Input: part model. Units: mm. Frame: model coordinates. A direction names the side the tool comes from. Coordinates: 2 decimals unless noted, no trailing zeros. Loops run counter-clockwise (first coordinate to the right, second up) from the corner with the lowest first, then second, coordinate; pieces in that order, holes last.
```python
from build123d import *

# Parameters (mm, degrees)
SKETCH_1_W          = 136
SKETCH_1_H          = 104
EXTRUDE_1_DEPTH     = 42
SKETCH_2_W          = 130
SKETCH_2_H          = 98
CUT_EXTRUDE_1_DEPTH = 36
CUT_EXTRUDE_2_REACH = 94.865
SKETCH_3_R          = 5
SKETCH_4_R          = 5
CUT_EXTRUDE_3_DEPTH = 136
SKETCH_5_R          = 5
CUT_EXTRUDE_4_DEPTH = 104
SKETCH_6_W          = 3
SKETCH_6_H          = 20
EXTRUDE_2_DEPTH     = 100
SKETCH_7_R          = 10
EXTRUDE_3_DEPTH     = 130
EXTRUDE_4_DEPTH     = 3
EXTRUDE_START       = -3
EXTRUDE_5_DEPTH     = 3
SKETCH_10_W         = 1.2
SKETCH_10_H         = 2
CUT_EXTRUDE_5_DEPTH = 104
SKETCH_11_W         = 1.2
SKETCH_11_H         = 2
CUT_EXTRUDE_6_DEPTH = 136


with BuildPart() as part:
    # 草图1 → 凸台-拉伸1 (new body)
    with BuildSketch(Plane(origin=(0, 0, 0), x_dir=(1, 0, 0), z_dir=(0, 1, 0))):
        Rectangle(SKETCH_1_W, SKETCH_1_H)
    extrude(amount=EXTRUDE_1_DEPTH)

    # 草图2 → 切除-拉伸1 (cut)
    with BuildSketch(Plane(origin=(0, 42, 0), x_dir=(1, 0, 0), z_dir=(0, 1, 0))):
        Rectangle(SKETCH_2_W, SKETCH_2_H)
    extrude(amount=-CUT_EXTRUDE_1_DEPTH, mode=Mode.SUBTRACT)

    # 草图3 → 切除-拉伸2 (cut, up to next)
    with BuildSketch(Plane(origin=(0, 6, 0), x_dir=(1, 0, 0), z_dir=(0, 1, 0)), mode=Mode.PRIVATE) as cut_extrude_2_sk1:
        with Locations(Location((-34, 26, 0), (0, 0, 270))):
            Circle(SKETCH_3_R)
    cut_extrude_2_tool1 = extrude(cut_extrude_2_sk1.sketch, amount=-CUT_EXTRUDE_2_REACH, mode=Mode.PRIVATE) & part.part
    # 草图3 → 切除-拉伸2 (cut, up to next)
    with BuildSketch(Plane(origin=(0, 6, 0), x_dir=(1, 0, 0), z_dir=(0, 1, 0)), mode=Mode.PRIVATE) as cut_extrude_2_sk2:
        with Locations(Location((-34, -26, 0), (0, 0, 270))):
            Circle(SKETCH_3_R)
    cut_extrude_2_tool2 = extrude(cut_extrude_2_sk2.sketch, amount=-CUT_EXTRUDE_2_REACH, mode=Mode.PRIVATE) & part.part
    # 草图3 → 切除-拉伸2 (cut, up to next)
    with BuildSketch(Plane(origin=(0, 6, 0), x_dir=(1, 0, 0), z_dir=(0, 1, 0)), mode=Mode.PRIVATE) as cut_extrude_2_sk3:
        with Locations(Location((34, 26, 0), (0, 0, 270))):
            Circle(SKETCH_3_R)
    cut_extrude_2_tool3 = extrude(cut_extrude_2_sk3.sketch, amount=-CUT_EXTRUDE_2_REACH, mode=Mode.PRIVATE) & part.part
    # 草图3 → 切除-拉伸2 (cut, up to next)
    with BuildSketch(Plane(origin=(0, 6, 0), x_dir=(1, 0, 0), z_dir=(0, 1, 0)), mode=Mode.PRIVATE) as cut_extrude_2_sk4:
        with Locations(Location((34, -26, 0), (0, 0, 270))):
            Circle(SKETCH_3_R)
    cut_extrude_2_tool4 = extrude(cut_extrude_2_sk4.sketch, amount=-CUT_EXTRUDE_2_REACH, mode=Mode.PRIVATE) & part.part
    # 草图3 → 切除-拉伸2 (cut, up to next)
    with BuildSketch(Plane(origin=(0, 6, 0), x_dir=(1, 0, 0), z_dir=(0, 1, 0)), mode=Mode.PRIVATE) as cut_extrude_2_sk5:
        with Locations(Location((0, 26, 0), (0, 0, 270))):
            Circle(SKETCH_3_R)
    cut_extrude_2_tool5 = extrude(cut_extrude_2_sk5.sketch, amount=-CUT_EXTRUDE_2_REACH, mode=Mode.PRIVATE) & part.part
    # 草图3 → 切除-拉伸2 (cut, up to next)
    with BuildSketch(Plane(origin=(0, 6, 0), x_dir=(1, 0, 0), z_dir=(0, 1, 0)), mode=Mode.PRIVATE) as cut_extrude_2_sk6:
        with Locations(Location((0, 0, 0), (0, 0, 270))):
            Circle(SKETCH_3_R)
    cut_extrude_2_tool6 = extrude(cut_extrude_2_sk6.sketch, amount=-CUT_EXTRUDE_2_REACH, mode=Mode.PRIVATE) & part.part
    # 草图3 → 切除-拉伸2 (cut, up to next)
    with BuildSketch(Plane(origin=(0, 6, 0), x_dir=(1, 0, 0), z_dir=(0, 1, 0)), mode=Mode.PRIVATE) as cut_extrude_2_sk7:
        with Locations(Location((-34, 0, 0), (0, 0, 270))):
            Circle(SKETCH_3_R)
    cut_extrude_2_tool7 = extrude(cut_extrude_2_sk7.sketch, amount=-CUT_EXTRUDE_2_REACH, mode=Mode.PRIVATE) & part.part
    # 草图3 → 切除-拉伸2 (cut, up to next)
    with BuildSketch(Plane(origin=(0, 6, 0), x_dir=(1, 0, 0), z_dir=(0, 1, 0)), mode=Mode.PRIVATE) as cut_extrude_2_sk8:
        with Locations(Location((0, -26, 0), (0, 0, 270))):
            Circle(SKETCH_3_R)
    cut_extrude_2_tool8 = extrude(cut_extrude_2_sk8.sketch, amount=-CUT_EXTRUDE_2_REACH, mode=Mode.PRIVATE) & part.part
    # 草图3 → 切除-拉伸2 (cut, up to next)
    with BuildSketch(Plane(origin=(0, 6, 0), x_dir=(1, 0, 0), z_dir=(0, 1, 0)), mode=Mode.PRIVATE) as cut_extrude_2_sk9:
        with Locations(Location((34, 0, 0), (0, 0, 270))):
            Circle(SKETCH_3_R)
    cut_extrude_2_tool9 = extrude(cut_extrude_2_sk9.sketch, amount=-CUT_EXTRUDE_2_REACH, mode=Mode.PRIVATE) & part.part
    add(cut_extrude_2_tool1.solids().sort_by_distance((-34, 6, -26))[0], mode=Mode.SUBTRACT)
    add(cut_extrude_2_tool2.solids().sort_by_distance((-34, 6, 26))[0], mode=Mode.SUBTRACT)
    add(cut_extrude_2_tool3.solids().sort_by_distance((34, 6, -26))[0], mode=Mode.SUBTRACT)
    add(cut_extrude_2_tool4.solids().sort_by_distance((34, 6, 26))[0], mode=Mode.SUBTRACT)
    add(cut_extrude_2_tool5.solids().sort_by_distance((0, 6, -26))[0], mode=Mode.SUBTRACT)
    add(cut_extrude_2_tool6.solids().sort_by_distance((0, 6, 0))[0], mode=Mode.SUBTRACT)
    add(cut_extrude_2_tool7.solids().sort_by_distance((-34, 6, 0))[0], mode=Mode.SUBTRACT)
    add(cut_extrude_2_tool8.solids().sort_by_distance((0, 6, 26))[0], mode=Mode.SUBTRACT)
    add(cut_extrude_2_tool9.solids().sort_by_distance((34, 6, 0))[0], mode=Mode.SUBTRACT)

    # 草图4 → 切除-拉伸3 (cut)
    with BuildSketch(Plane.ZY.offset(68)):
        with Locations((-25, 21)):
            Circle(SKETCH_4_R)
        with Locations((25, 21)):
            Circle(SKETCH_4_R)
    extrude(amount=-CUT_EXTRUDE_3_DEPTH, mode=Mode.SUBTRACT)

    # 草图5 → 切除-拉伸4 (cut)
    with BuildSketch(Plane.XY.offset(52)):
        with Locations((-34, 21)):
            Circle(SKETCH_5_R)
        with Locations((34, 21)):
            Circle(SKETCH_5_R)
        with Locations((0, 21)):
            Circle(SKETCH_5_R)
    extrude(amount=-CUT_EXTRUDE_4_DEPTH, mode=Mode.SUBTRACT)

    # 草图6 → 凸台-拉伸2 (add)
    with BuildSketch(Plane(origin=(0, 42, 0), x_dir=(1, 0, 0), z_dir=(0, 1, 0))):
        with Locations((-66.5, 0)):
            Rectangle(SKETCH_6_W, SKETCH_6_H)
        with Locations((66.5, 0)):
            Rectangle(SKETCH_6_W, SKETCH_6_H)
    extrude(amount=EXTRUDE_2_DEPTH)

    # 草图7 → 凸台-拉伸3 (add)
    with BuildSketch(Plane(origin=(-65, 0, 0), x_dir=(0, 0, -1), z_dir=(1, 0, 0))):
        with Locations(Location((0, 142, 0), (0, 0, 180))):
            Circle(SKETCH_7_R)
    extrude(amount=EXTRUDE_3_DEPTH)

    # 草图8 → 凸台-拉伸4 (add)
    with BuildSketch(Plane.ZY.offset(68)):
        with BuildLine():
            Line((-10, 142), (10, 142))
            ThreePointArc((10, 142), (0, 152), (-10, 142))
        make_face()
    extrude(amount=-EXTRUDE_4_DEPTH)

    # 草图9 → 凸台-拉伸5 (add)
    with BuildSketch(Plane(origin=(68, 0, 0), x_dir=(0, 0, -1), z_dir=(1, 0, 0)).offset(EXTRUDE_START)):
        with BuildLine():
            Line((-10, 142), (10, 142))
            ThreePointArc((10, 142), (0, 152), (-10, 142))
        make_face()
    extrude(amount=EXTRUDE_5_DEPTH)

    # 草图10 → 切除-拉伸5 (cut)
    with BuildSketch(Plane.XY.offset(52)):
        with Locations((-34, 42)):
            Rectangle(SKETCH_10_W, SKETCH_10_H)
        with Locations((34, 42)):
            Rectangle(SKETCH_10_W, SKETCH_10_H)
    extrude(amount=-CUT_EXTRUDE_5_DEPTH, mode=Mode.SUBTRACT)

    # 草图11 → 切除-拉伸6 (cut)
    with BuildSketch(Plane.ZY.offset(68)):
        with Locations((-25, 42)):
            Rectangle(SKETCH_11_W, SKETCH_11_H)
        with Locations((25, 42)):
            Rectangle(SKETCH_11_W, SKETCH_11_H)
    extrude(amount=-CUT_EXTRUDE_6_DEPTH, mode=Mode.SUBTRACT)


solid = part.part
```
Item 1: Contact query for flat-ended pins moving along their axis: P1, Ø11.5, axis at x = -34, z = 26, coming from the +Y side; P2, Ø3.5, axis at x = 66.5, z = 15, coming from the +Y side; P3, Ø1.5, axis at x = -66, y = 87, coming from the -Z side. Output: stop coordinate, or through.
Result:
P1: stops at y = 6
P2: stops at y = 42
P3: stops at z = -10
Item 2: Section query B-B (x = 9). Output: boundary loops of the cut face in (y, z).
Result:
outline: (0, -52) - (42, -52) - (42, -49) - (6, -49) - (6, 49) - (42, 49) - (42, 52) - (0, 52) - close; circle Ø20 at (142, 0)
Item 3: Line query: L1, parallel to X at y = 1.45, z = -26; L2, parallel to X at y = 30, z = 32; L3, parallel to Z at x = -11, y = 19. Output: solid intervals per line, ascending.
Result:
L1: x = -68 to -39, -29 to -5, 5 to 29, 39 to 68
L2: x = -68 to -65, 65 to 68
L3: z = -52 to -49, 49 to 52
Item 4: Section query D-D (z = 27.5). Output: boundary loops of the cut face in (x, y).
Result:
outline: (-68, 0) - (-38.77, 0) - (-38.77, 6) - (-65, 6) - (-65, 16.67) - (-68, 16.67) - close; (-68, 25.33) - (-65, 25.33) - (-65, 42) - (-68, 42) - close; (-29.23, 0) - (-4.77, 0) - (-4.77, 6) - (-29.23, 6) - close; (4.77, 0) - (29.23, 0) - (29.23, 6) - (4.77, 6) - close; (38.77, 0) - (68, 0) - (68, 16.67) - (65, 16.67) - (65, 6) - (38.77, 6) - close; (65, 25.33) - (68, 25.33) - (68, 42) - (65, 42) - close
Item 5: Mould query, pull axis Y, two halves, no side actions, for faces 1 (the face through (-59, 42, -50)), 2 (the face through (-38, 18, -50)), 3 (the face through (-1, 28, -49)), 4 (the face through (-66.52, 16.12, 23.92)). Classes: +Y half, -Y half, draft (parallel to the pull), parting line (faces both ways), or undercut.
Result:
face 1: +Y half
face 2: undercut
face 3: draft
face 4: undercut
Item 6: Section query C-C (y = 127). Output: boundary loops of the cut face in (x, z).
Result:
outline: (-68, -10) - (-65, -10) - (-65, 10) - (-68, 10) - close; (65, -10) - (68, -10) - (68, 10) - (65, 10) - close
Item 7: Reachability of faces 5 (the face through (57, 42, -50)), 6 (the face through (-38.88, 3.04, -1.08)), 7 (the face through (-57.6, 42, 49.5)), 8 (the face through (-1, 28, 49)) from +Z, -Z, +X, -X, +Y, -Y: full face, straight path, thin tool, end or side. Return the list, or none.
Result:
face 5: -Z, +X, -X, +Y
face 6: -Y
face 7: +Z, +X, -X, +Y
face 8: +Y
Item 8: Section query A-A (z = 0). Output: boundary loops of the cut face in (x, y).
Result:
outline: (-68, 0) - (-39, 0) - (-39, 6) - (-65, 6) - (-65, 132) - (65, 132) - (65, 6) - (39, 6) - (39, 0) - (68, 0) - (68, 152) - (-68, 152) - close; (-29, 0) - (-5, 0) - (-5, 6) - (-29, 6) - close; (5, 0) - (29, 0) - (29, 6) - (5, 6) - close
